```python
from build123d import *

# Parameters (mm, degrees)
SKETCH1_W           = 67
SKETCH1_H           = 155
SKETCH1_W_2         = 160
SKETCH1_H_2         = 110
SKETCH1_W_3         = 18.62
SKETCH1_H_3         = 29.1
BOSS_EXTRUDE1_DEPTH = 5
SKETCH4_W           = 100
SKETCH4_H           = 2
BOSS_EXTRUDE2_DEPTH = 10
SKETCH9_W           = 0.845761127
SKETCH9_H           = 22.5
BOSS_EXTRUDE4_DEPTH = 5
BOSS_EXTRUDE3_DEPTH = 5
SKETCH7_R           = 2.05
CUT_EXTRUDE2_DEPTH  = 10
SKETCH6_R           = 2.05
CUT_EXTRUDE1_DEPTH  = 227.055622359
SKETCH10_R          = 2.05
CUT_EXTRUDE4_DEPTH  = 10
FILLET1_R           = 0.3
SKETCH16_R          = 2.05
CUT_EXTRUDE5_DEPTH  = 251.551680098
SKETCH18_W          = 4
SKETCH18_H          = 2.5
BOSS_EXTRUDE7_DEPTH = 7
SKETCH20_W          = 4.2
SKETCH20_H          = 2.7
SKETCH20_W_2        = 4
SKETCH20_H_2        = 2.5
CUT_EXTRUDE7_DEPTH  = 8
SKETCH21_W          = 4
SKETCH21_H          = 2.5
CUT_EXTRUDE8_DEPTH  = 1


with BuildPart() as part:
    # Sketch1 → Boss-Extrude1 (new body)
    with BuildSketch(Plane(origin=(0, 0, 0), x_dir=(1, 0, 0), z_dir=(0, 1, 0))):
        Rectangle(SKETCH1_W, SKETCH1_H)
        with Locations((-113.5, 0)):
            Rectangle(SKETCH1_W_2, SKETCH1_H_2)
        with Locations((-202.81, 0)):
            Rectangle(SKETCH1_W_3, SKETCH1_H_3)
    extrude(amount=BOSS_EXTRUDE1_DEPTH)

    # Sketch4 → Boss-Extrude2 (add)
    with BuildSketch(Plane(origin=(0, 5, 0), x_dir=(1, 0, 0), z_dir=(0, 1, 0))):
        with Locations((-143.5, -54)):
            Rectangle(SKETCH4_W, SKETCH4_H)
        with Locations((-143.5, 54)):
            Rectangle(SKETCH4_W, SKETCH4_H)
    extrude(amount=BOSS_EXTRUDE2_DEPTH)

    # Sketch9 → Boss-Extrude4 (add)
    with BuildSketch(Plane(origin=(0, 5, 0), x_dir=(1, 0, 0), z_dir=(0, 1, 0))):
        with Locations((-33.922880564, -66.25)):
            Rectangle(SKETCH9_W, SKETCH9_H)
        with Locations((-33.922880564, 66.25)):
            Rectangle(SKETCH9_W, SKETCH9_H)
    extrude(amount=-BOSS_EXTRUDE4_DEPTH)

    # Sketch5 → Boss-Extrude3 (add)
    with BuildSketch(Plane(origin=(0, 5, 0), x_dir=(1, 0, 0), z_dir=(0, 1, 0))):
        Polygon((-178, 27), (-172.5, 27), (-172.5, 34.2), (-183.5, 34.2), (-183.5, 19.3), (-178, 19.3), align=None)
        Polygon((-178, -27.15), (-172.5, -27.15), (-172.5, -34.35), (-183.5, -34.35), (-183.5, -19.45), (-178, -19.45), align=None)
        Polygon((-13.85, 27), (-13.85, 19.3), (-8.35, 19.3), (-8.35, 34.2), (-19.35, 34.2), (-19.35, 27), align=None)
        Polygon((-19.35, -27.15), (-19.35, -34.35), (-8.35, -34.35), (-8.35, -19.45), (-13.85, -19.45), (-13.85, -27.15), align=None)
    extrude(amount=BOSS_EXTRUDE3_DEPTH)

    # Sketch7 → Cut-Extrude2 (cut)
    with BuildSketch(Plane(origin=(0, 5, 0), x_dir=(1, 0, 0), z_dir=(0, 1, 0))):
        with Locations(Location((-207.12, 10.268043156, 0), (0, 0, 270))):
            Circle(SKETCH7_R)
        with Locations(Location((-207.12, -9.741956844, 0), (0, 0, 270))):
            Circle(SKETCH7_R)
    extrude(amount=-CUT_EXTRUDE2_DEPTH, mode=Mode.SUBTRACT)

    # Sketch6 → Cut-Extrude1 (cut, through all)
    with BuildSketch(Plane(origin=(0, 5, 0), x_dir=(1, 0, 0), z_dir=(0, 1, 0))):
        with Locations(Location((-85.880982052, -48, 0), (0, 0, 270))):
            Circle(SKETCH6_R)
        with Locations(Location((-57.380982052, -48, 0), (0, 0, 270))):
            Circle(SKETCH6_R)
        with Locations(Location((-57.380982052, 48, 0), (0, 0, 90))):
            Circle(SKETCH6_R)
        with Locations(Location((-85.880982052, 48, 0), (0, 0, 90))):
            Circle(SKETCH6_R)
    extrude(amount=-CUT_EXTRUDE1_DEPTH, mode=Mode.SUBTRACT)

    # Sketch10 → Cut-Extrude4 (cut)
    with BuildSketch(Plane(origin=(0, 5, 0), x_dir=(1, 0, 0), z_dir=(0, 1, 0))):
        with Locations(Location((-183.5, 44.599757133, 0), (0, 0, 270))):
            Circle(SKETCH10_R)
        with Locations(Location((-137.5, 44.599757133, 0), (0, 0, 270))):
            Circle(SKETCH10_R)
        with Locations(Location((-183.5, -43.400242867, 0), (0, 0, 270))):
            Circle(SKETCH10_R)
        with Locations(Location((-137.5, -43.400242867, 0), (0, 0, 270))):
            Circle(SKETCH10_R)
    extrude(amount=-CUT_EXTRUDE4_DEPTH, mode=Mode.SUBTRACT)

    # Fillet1
    fillet1_edges = [part.edges().sort_by_distance(p)[0] for p in [
        (-34.345761127, 2.5, 55),
        (-34.345761127, 2.5, -55),
    ]]
    fillet(fillet1_edges, radius=FILLET1_R)

    # Sketch16 → Cut-Extrude5 (cut, through all)
    with BuildSketch(Plane.XY.offset(55)):
        with Locations((-140.228178999, 10)):
            Circle(SKETCH16_R)
        with Locations((-125.228178999, 10)):
            Circle(SKETCH16_R)
        with Locations((-110.228178999, 10)):
            Circle(SKETCH16_R)
        with Locations((-155.228178999, 10)):
            Circle(SKETCH16_R)
        with Locations((-170.228178999, 10)):
            Circle(SKETCH16_R)
        with Locations((-185.228178999, 10)):
            Circle(SKETCH16_R)
    extrude(amount=-CUT_EXTRUDE5_DEPTH, mode=Mode.SUBTRACT)


with BuildPart() as body_2:
    # Split1: the piece on the far side of the plane
    add(part.part)
    split(bisect_by=Plane(origin=(-34.345761127, 0, 0), x_dir=(0, 0, 1), z_dir=(1, 0, 0)), keep=Keep.BOTTOM)


with BuildPart() as part_1:
    add(part.part)

    # Split1
    split(bisect_by=Plane(origin=(-34.345761127, 0, 0), x_dir=(0, 0, 1), z_dir=(1, 0, 0)), keep=Keep.TOP)

    # Sketch18 → Boss-Extrude7 (add)
    with BuildSketch(Plane.ZY.offset(34.345761127)):
        with Locations((-39.5, 2.443337799)):
            Rectangle(SKETCH18_W, SKETCH18_H)
        with Locations((39.5, 2.443337799)):
            Rectangle(SKETCH18_W, SKETCH18_H)
    extrude(amount=BOSS_EXTRUDE7_DEPTH)


with BuildPart() as body_2_1:
    add(body_2.part)

    # Combine1: cut part
    add(part_1.part, mode=Mode.SUBTRACT)

    # Sketch20 → Cut-Extrude7 (cut)
    # profile 1 of 2: a face of its own
    with BuildSketch(Plane(origin=(-34.345761127, 0, 0), x_dir=(0, 0, -1), z_dir=(1, 0, 0))):
        with Locations((-39.5, 2.443337799)):
            Rectangle(SKETCH20_W, SKETCH20_H)
        with Locations((-39.5, 2.443337799)):
            Rectangle(SKETCH20_W_2, SKETCH20_H_2, mode=Mode.SUBTRACT)
    # profile 2 of 2: a face of its own
    with BuildSketch(Plane(origin=(-34.345761127, 0, 0), x_dir=(0, 0, -1), z_dir=(1, 0, 0))):
        with Locations((39.5, 2.443337799)):
            Rectangle(SKETCH20_W, SKETCH20_H)
        with Locations((39.5, 2.443337799)):
            Rectangle(SKETCH20_W_2, SKETCH20_H_2, mode=Mode.SUBTRACT)
    extrude(amount=-CUT_EXTRUDE7_DEPTH, mode=Mode.SUBTRACT)

    # Sketch21 → Cut-Extrude8 (cut)
    with BuildSketch(Plane(origin=(-41.345761127, 0, 0), x_dir=(0, 0, -1), z_dir=(1, 0, 0))):
        with Locations((39.5, 2.443337799)):
            Rectangle(SKETCH21_W, SKETCH21_H)
        with Locations((-39.5, 2.443337799)):
            Rectangle(SKETCH21_W, SKETCH21_H)
    extrude(amount=-CUT_EXTRUDE8_DEPTH, mode=Mode.SUBTRACT)


solid = body_2_1.part
```
Source: CAD feature listing. Evaluate the final solid. Frame: model axes, mm. A direction names the side the tool comes from. Round coordinates to 2 decimals unless told otherwise and drop trailing zeros. Loops run counter-clockwise (first coordinate to the right, second up) from the corner with the lowest first, then second, coordinate; pieces in that order, holes last. Notation, with made-up numbers: M 69.25,85.5 L 127.25,85.5 A20 ccw 127.25,98.5 Z; hole C 57.5,-10 d4. An arc over 180 degrees is marked long. Put each result on its own line as item: value.
(1) Ray query, line 1 (Z direction, x = -137.5, y = 1.25); line 2 (Z direction, x = -136, y = 14); line 3 (Y direction, x = -113, z = -19). Return the intervals inside material, ascending. Write a range as [from, to].
Solutions:
line 1: [-55, -46.65], [-42.55, 41.35], [45.45, 55]
line 2: [-55, -53], [53, 55]
line 3: [0, 5]
(2) Access query for faces 1 (the face through (-175, 7, -27)), 2 (the face through (-179, 10, -29)), 3 (the face through (-135.467, 2.535, -44.867)), 4 (the face through (-38, 1.093, 40)), 5 (the face through (-203, 2, 14.55)). Directions: +Z, -Z, +X, -X, +Y, -Y. A direction counts if a zero-diameter tool reaches every point of the face in a straight line with its end or side. Return the directions, or none.
Solutions:
face 1: +X, +Y
face 2: +X, -X, +Y
face 3: +Y, -Y
face 4: +X
face 5: +Z, -X, +Y, -Y
(3) First-contact query: pin 1 (3.5 mm diameter, centred on x = -125.23, y = 10, fed in from +Z); pin 2 (5.5 mm diameter, centred on x = -155.23, y = 10, fed in from -Z); pin 3 (4.5 mm diameter, centred on y = 6, z = -25.5, fed in from -X); pin 4 (2.5 mm diameter, centred on y = 8, z = 32, fed in from +X). Flat tips, straight axial feed; report the tip coordinate or a pass-through.
Solutions:
pin 1: through
pin 2: z = -55
pin 3: x = -193.5
pin 4: x = -172.5
(4) Section A-A, the plane x = -207.12. Return loops of the section in (y, z), and give its area (4 significant figures).
Solutions:
outline: M 0,-14.55 L 5,-14.55 L 5,-12.32 L 0,-12.32 Z; M 0,-8.22 L 5,-8.22 L 5,7.69 L 0,7.69 Z; M 0,11.79 L 5,11.79 L 5,14.55 L 0,14.55 Z
area: 104.5 mm²
(5) Section B-B, the plane x = -99.5. Return loops of the section in (y, z), and give its area (3 significant figures).
Solutions:
outline: M 0,-55 L 15,-55 L 15,-53 L 5,-53 L 5,53 L 15,53 L 15,55 L 0,55 Z
area: 590 mm²
(6) Pull-direction query (X, two-part tool) for faces 6 (the face through (-193.5, 4, -36)), 7 (the face through (-178, 7, -23)), 8 (the face through (-85.97, 2.54, -45.95)); classes: released by +X, released by -X, zero draft, split by the parting line, or undercut.
Solutions:
face 6: released by -X
face 7: released by +X
face 8: undercut
(7) Section D-D, the plane x = -62.5. Return loops of the section in (y, z).
Solutions:
outline: M 0,-55 L 5,-55 L 5,55 L 0,55 Z
(8) Section C-C, the plane z = 4. Return loops of the section in (x, y), and give its area (3 significant figures).
Solutions:
outline: M -212.12,0 L -34.35,0 L -34.35,5 L -212.12,5 Z
area: 889 mm²
